from build123d import *

# Parameters (mm, degrees)
F0_W     = 800
F0_H     = 100
F1_DEPTH = 800
F2_W     = 18
F2_H     = 5
F3_DEPTH = 800


with BuildPart() as f1:
    # F0 (on Top) → F1 (new body)
    with BuildSketch(Plane.XY):
        with Locations((400, 50)):
            Rectangle(F0_W, F0_H)
    extrude(amount=F1_DEPTH)

    # F2 (on face) → F3 (cut, through all)
    with BuildSketch(Plane.XY.offset(800)):
        Polygon((30, 50), (30, 20), (773, 20), (773, 50), (773, 80), (30, 80), align=None)
        with Locations((39, 2.5)):
            Rectangle(F2_W, F2_H)
        with Locations((64, 2.5)):
            Rectangle(F2_W, F2_H)
        with Locations((89, 2.5)):
            Rectangle(F2_W, F2_H)
        with Locations((114, 2.5)):
            Rectangle(F2_W, F2_H)
        with Locations((139, 2.5)):
            Rectangle(F2_W, F2_H)
        with Locations((339, 97.5)):
            Rectangle(F2_W, F2_H)
        with Locations((289, 2.5)):
            Rectangle(F2_W, F2_H)
        with Locations((264, 2.5)):
            Rectangle(F2_W, F2_H)
        with Locations((239, 2.5)):
            Rectangle(F2_W, F2_H)
        with Locations((689, 97.5)):
            Rectangle(F2_W, F2_H)
        with Locations((364, 97.5)):
            Rectangle(F2_W, F2_H)
        with Locations((639, 2.5)):
            Rectangle(F2_W, F2_H)
        with Locations((614, 2.5)):
            Rectangle(F2_W, F2_H)
        with Locations((589, 2.5)):
            Rectangle(F2_W, F2_H)
        with Locations((314, 97.5)):
            Rectangle(F2_W, F2_H)
        with Locations((664, 97.5)):
            Rectangle(F2_W, F2_H)
        with Locations((539, 2.5)):
            Rectangle(F2_W, F2_H)
        with Locations((514, 97.5)):
            Rectangle(F2_W, F2_H)
        with Locations((314, 2.5)):
            Rectangle(F2_W, F2_H)
        with Locations((214, 2.5)):
            Rectangle(F2_W, F2_H)
        with Locations((189, 2.5)):
            Rectangle(F2_W, F2_H)
        with Locations((164, 2.5)):
            Rectangle(F2_W, F2_H)
        with Locations((364, 2.5)):
            Rectangle(F2_W, F2_H)
        with Locations((339, 2.5)):
            Rectangle(F2_W, F2_H)
        with Locations((389, 2.5)):
            Rectangle(F2_W, F2_H)
        with Locations((714, 2.5)):
            Rectangle(F2_W, F2_H)
        with Locations((614, 97.5)):
            Rectangle(F2_W, F2_H)
        with Locations((514, 2.5)):
            Rectangle(F2_W, F2_H)
        with Locations((214, 97.5)):
            Rectangle(F2_W, F2_H)
        with Locations((114, 97.5)):
            Rectangle(F2_W, F2_H)
        with Locations((489, 2.5)):
            Rectangle(F2_W, F2_H)
        with Locations((89, 97.5)):
            Rectangle(F2_W, F2_H)
        with Locations((714, 97.5)):
            Rectangle(F2_W, F2_H)
        with Locations((464, 2.5)):
            Rectangle(F2_W, F2_H)
        with Locations((189, 97.5)):
            Rectangle(F2_W, F2_H)
        with Locations((689, 2.5)):
            Rectangle(F2_W, F2_H)
        with Locations((439, 97.5)):
            Rectangle(F2_W, F2_H)
        with Locations((289, 97.5)):
            Rectangle(F2_W, F2_H)
        with Locations((439, 2.5)):
            Rectangle(F2_W, F2_H)
        with Locations((264, 97.5)):
            Rectangle(F2_W, F2_H)
        with Locations((389, 97.5)):
            Rectangle(F2_W, F2_H)
        with Locations((664, 2.5)):
            Rectangle(F2_W, F2_H)
        with Locations((464, 97.5)):
            Rectangle(F2_W, F2_H)
        with Locations((414, 2.5)):
            Rectangle(F2_W, F2_H)
        with Locations((539, 97.5)):
            Rectangle(F2_W, F2_H)
        with Locations((564, 97.5)):
            Rectangle(F2_W, F2_H)
        with Locations((639, 97.5)):
            Rectangle(F2_W, F2_H)
        with Locations((164, 97.5)):
            Rectangle(F2_W, F2_H)
        with Locations((139, 97.5)):
            Rectangle(F2_W, F2_H)
        with Locations((39, 97.5)):
            Rectangle(F2_W, F2_H)
        with Locations((564, 2.5)):
            Rectangle(F2_W, F2_H)
        with Locations((239, 97.5)):
            Rectangle(F2_W, F2_H)
        with Locations((414, 97.5)):
            Rectangle(F2_W, F2_H)
        with Locations((589, 97.5)):
            Rectangle(F2_W, F2_H)
        with Locations((764, 2.5)):
            Rectangle(F2_W, F2_H)
        with Locations((64, 97.5)):
            Rectangle(F2_W, F2_H)
        with Locations((739, 2.5)):
            Rectangle(F2_W, F2_H)
        with Locations((489, 97.5)):
            Rectangle(F2_W, F2_H)
        with Locations((739, 97.5)):
            Rectangle(F2_W, F2_H)
        with Locations((764, 97.5)):
            Rectangle(F2_W, F2_H)
    extrude(amount=-F3_DEPTH, mode=Mode.SUBTRACT)


solid = f1.part
Work out the finished part from the listing and answer in its coordinate system (mm). A direction names the side the tool comes from. Round coordinates to 2 decimals unless told otherwise and drop trailing zeros. Loops run counter-clockwise (first coordinate to the right, second up) from the corner with the lowest first, then second, coordinate; pieces in that order, holes last. Notation, with made-up numbers: (29.5, 46) - (33.5, 46) arc R7 cw to (33.5, 54) - close; hole circle Ø7 at (-4, 50). An arc over 180 degrees is marked (long way). Use one line per item in the form item = value. Start each with the question number.
(1) Flat-ended cylindrical pins translate along their axes: P1, Ø5.5, axis at x = 762, z = 449, coming from the -Y side; P2, Ø10, axis at x = 424.5, z = 230.5, coming from the -Y side; P3, Ø9, axis at x = 288, z = 461.5, coming from the +Y side. Find the tip coordinate at first contact, or state that the pin passes through.
(2) Which of the six approach directions +Z, -Z, +X, -X, +Y, -Y give full straight-line access (tool end or side, diameter ignored) to faces 3 (the face through (739, 95, 406)), 4 (the face through (398, 13, 800)), 5 (the face through (189, 5, 406))?
(3) Find section A-A on y = 34.5. Determine the outline of the cut face in (x, z), and give its area (3 significant figures).
(4) Determine the mould class of faces 1 (the face through (15, 100, 394)), 2 (the face through (189, 95, 406)) for opening direction X: +X half, -X half, draft (parallel to the pull), parting line (faces both ways), or undercut.
(5) Consider line 1 (Y direction, x = 677, z = 198); line 2 (X direction, y = 22, z = 344.5); line 3 (Y direction, x = 258.5, z = 259.5). Determine where each line is inside the solid, lowest interval first.
Answer list:
q1.P1 = 5
q1.P2 = 0
q1.P3 = 95
q2.face_3 = +Z, -Z, +Y
q2.face_4 = +Z, +X, -X, +Y, -Y
q2.face_5 = +Z, -Z, -Y
q3.outline = (0, 0) - (30, 0) - (30, 800) - (0, 800) - close; (773, 0) - (800, 0) - (800, 800) - (773, 800) - close
q3.area = 45,600 mm^2
q4.face_1 = draft
q4.face_2 = undercut
q5.line_1 = 0 to 20, 80 to 100
q5.line_2 = 0 to 30, 773 to 800
q5.line_3 = 5 to 20, 80 to 95
